Read the model definition and answer for the solid it produces. Units are mm, in the model's axes. Face numbers are marked on the shaded views. A direction names the side the tool comes from. Coordinates: 2 decimals unless noted, no trailing zeros. Write each loop counter-clockwise with the first axis right and the second up, starting at its lowest first coordinate (ties: lowest second). Pieces come first, ordered by that corner, then holes. Notation, with made-up numbers: (36.25, -15) - (75.25, -15) arc R32 ccw to (75.25, 19) - close; hole circle Ø1 at (47, 40.25). An arc over 180 degrees is marked (long way). Use a Markdown table: item, result.
from build123d import *

# Parameters (mm, degrees)
F0_W           = 150
F0_H           = 150
F1_DEPTH       = 6
F1_DEPTH_BACK  = 6
F3_D           = 11
F3_CSINK_D     = 22.4
F3_CSINK_ANGLE = 90
F4_W           = 65
F4_H           = 65
F5_DEPTH       = 120
F6_T           = -7.5


with BuildPart() as f1:
    # F0 (on Top) → F1 (new body, two sides)
    with BuildSketch(Plane.XY) as f1_sk:
        Rectangle(F0_W, F0_H)
    extrude(amount=F1_DEPTH)
    extrude(f1_sk.sketch, amount=-F1_DEPTH_BACK)

    # F3 (through all)
    with Locations(Plane.XY.offset(6)):
        with Locations((-51, 51), (51, 51), (51, -51), (-51, -51)):
            CounterSinkHole(F3_D / 2, F3_CSINK_D / 2, counter_sink_angle=F3_CSINK_ANGLE)

    # F4 (on face) → F5 (join)
    with BuildSketch(Plane(origin=(0, 0, -6), x_dir=(1, 0, 0), z_dir=(0, 0, -1))):
        Rectangle(F4_W, F4_H)
    extrude(amount=F5_DEPTH)

    # F6
    f6_openings = [f1.faces().sort_by_distance(p)[0] for p in [
        (0, 0, -126),
    ]]
    offset(amount=F6_T, openings=f6_openings, kind=Kind.INTERSECTION)


solid = f1.part
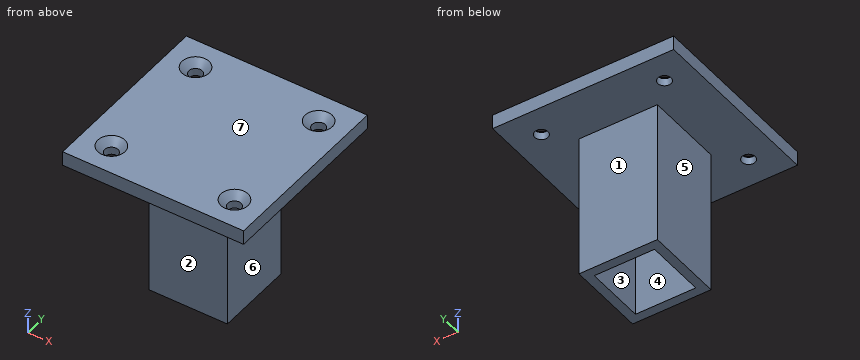
(1) Each of these flat-tipped pins is pushed along its axis until it touches: P1, Ø15, axis at x = 4, z = -76.5, coming from the -Y side; P2, Ø1, axis at x = 25, z = -22, coming from the +Y side; P3, Ø8, axis at x = -55.5, y = 1, coming from the -Z side. Where does it stop, or does it pass through?
Report:
| item | result |
|---|---|
| P1 | stops at y = -32.5 |
| P2 | stops at y = 32.5 |
| P3 | stops at z = -6 |
(2) The mould has two halves that part along Y. Classify the marked faces 1, 2, 3 and 4: pulls with the +Y half, pulls with the -Y half, needs draft (parallel to the pull), parting line crosses it, or undercut.
Report:
| item | result |
|---|---|
| face 1 | pulls with the +Y half |
| face 2 | pulls with the -Y half |
| face 3 | undercut |
| face 4 | undercut |
(3) A cutting plane is placed at D-D, the plane x = 20. Write down the section's boundary in (y, z), and give its area (4 significant figures).
Report:
| item | result |
|---|---|
| outline | (-75, -6) - (-32.5, -6) - (-32.5, -126) - (-25, -126) - (-25, -1.5) - (25, -1.5) - (25, -126) - (32.5, -126) - (32.5, -6) - (75, -6) - (75, 6) - (-75, 6) - close |
| area | 3,375 mm² |
(4) Straight lines are drawn through the part: L1, parallel to Y at x = 51, z = -4; L2, parallel to Y at x = -3, z = -77.5. For each, find the intervals that lie inside material, in ascending order.
Report:
| item | result |
|---|---|
| L1 | y = -75 to -56.5, -45.5 to 45.5, 56.5 to 75 |
| L2 | y = -32.5 to -25, 25 to 32.5 |
(5) A cutting plane is placed at C-C, the plane z = -52.5. Write down the section's boundary in (x, y).
Report:
| item | result |
|---|---|
| outline | (-32.5, -32.5) - (32.5, -32.5) - (32.5, 32.5) - (-32.5, 32.5) - close; hole (-25, -25) - (25, -25) - (25, 25) - (-25, 25) - close |
(6) For the marked faces 5, 6 and 7, determine the directions among +Z, -Z, +X, -X, +Y, -Y from which every point of the face is accessible in a straight line to the end or side of a thin tool.
Report:
| item | result |
|---|---|
| face 5 | -Z, -X, +Y, -Y |
| face 6 | -Z, +X, +Y, -Y |
| face 7 | +Z, +X, -X, +Y, -Y |
(7) A cutting plane is placed at A-A, the plane y = 51. Write down the section's boundary in (x, z), and give its area (3 significant figures).
Report:
| item | result |
|---|---|
| outline | (-75, -6) - (-56.5, -6) - (-56.5, 0.3) - (-62.2, 6) - (-75, 6) - close; (-45.5, -6) - (45.5, -6) - (45.5, 0.3) - (39.8, 6) - (-39.8, 6) - (-45.5, 0.3) - close; (56.5, -6) - (75, -6) - (75, 6) - (62.2, 6) - (56.5, 0.3) - close |
| area | 1,470 mm² |
